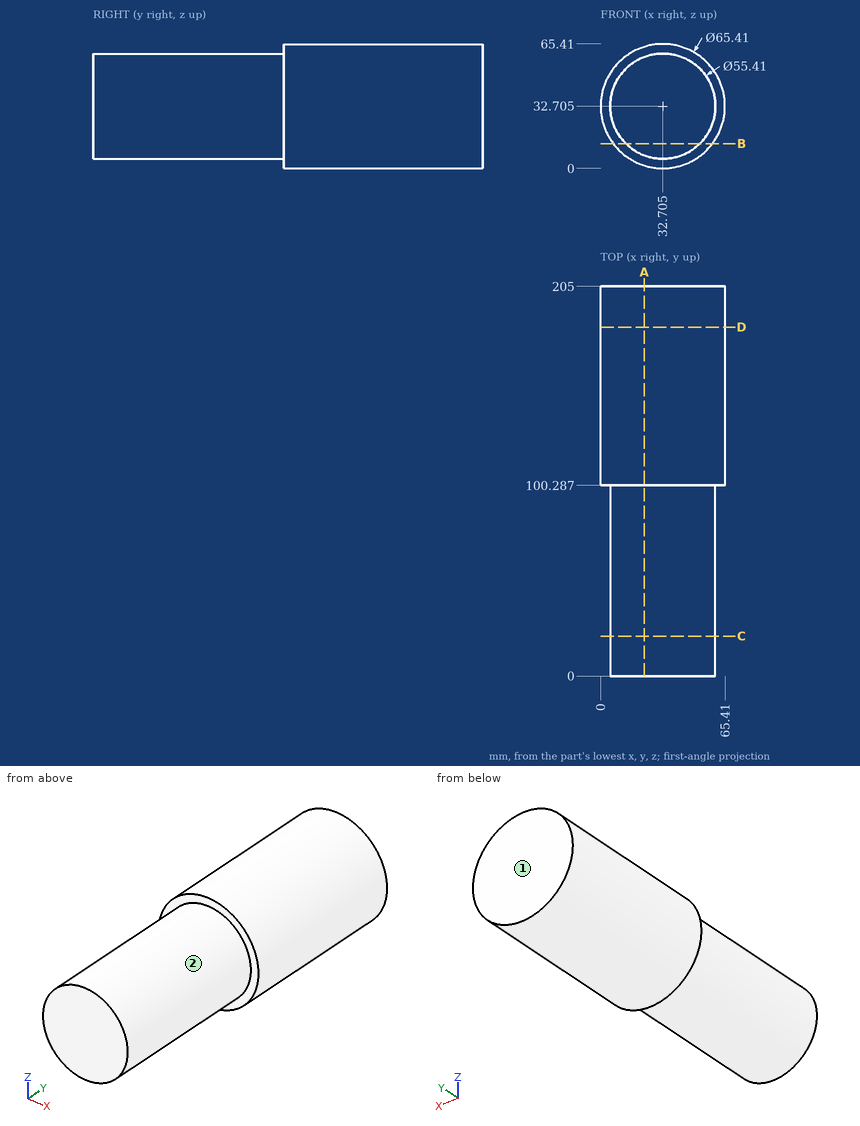
Study the drawing (mm; zero at the part's minimum x, y, z) and answer. A direction names the side the tool comes from. Round coordinates to 2 decimals unless told otherwise and drop trailing zeros. Write each loop counter-clockwise with the first axis right and the second up, starting at its lowest first coordinate (ties: lowest second). Pieces come first, ordered by that corner, then holes. Notation, with made-up numbers: (18, 27.25) - (39, 27.25) arc R13 cw to (39, 44.25) - close; hole circle Ø10 at (-37.5, 62). An arc over 180 degrees is marked (long way). Return JSON: item names as keys, results as strings. Group by question number.
Q1. The part is cut by section D-D on y = 183.5. Write down the section's boundary in (x, z) (3 decimals), then the cut area to 3 significant figures.
Q2. The part is cut by section B-B on z = 13. Write down the section's boundary in (x, y).
Q3. Each of these flat-tipped pins is pushed along its axis until it touches: pin 1 Ø4 at (y, z) = (46, 56.5) entering from -X; pin 2 Ø1 at (y, z) = (34, 58) entering from +X (1 decimal); pin 3 Ø5 at (x, y) = (20, 179.5) entering from +Z. Where does it stop, or does it pass through?
Q4. For the marked faces 1 and 2, determine the directions among +Z, -Z, +X, -X, +Y, -Y from which every point of the face is accessible in a straight line to the end or side of a thin tool.
Q5. The part is cut by section A-A on x = 23. Write down the section's boundary in (y, z), then the cut area to 3 significant figures.
Q6. Find the intervals of material crossed by L1, parallel to Z at x = 31.5, y = 125; L2, parallel to Y at x = 53, z = 54; L3, parallel to X at y = 191, z = 32, in increasing order.
Q7. The part is cut by section C-C on y = 21. Write down the section's boundary in (x, z) (3 decimals).
Solved:
{
 "1": {"outline": "circle Ø65.41 at (32.705, 32.705)", "area": "3,360 mm²"},
 "2": {"outline": "(6.6, 100.29) - (13.23, 100.29) - (13.23, 0) - (52.18, 0) - (52.18, 100.29) - (58.81, 100.29) - (58.81, 205) - (6.6, 205) - close"},
 "3": {"pin 1": "x = 15.6", "pin 2": "x = 45.1", "pin 3": "z = 63.78"},
 "4": {"face 1": "+Z, -Z, +X, -X, +Y", "face 2": "-Y"},
 "5": {"outline": "(0, 6.76) - (100.29, 6.76) - (100.29, 1.47) - (205, 1.47) - (205, 63.94) - (100.29, 63.94) - (100.29, 58.65) - (0, 58.65) - close", "area": "11,700 mm²"},
 "6": {"L1": "0.02 to 65.39", "L2": "100.29 to 205", "L3": "0.01 to 65.4"},
 "7": {"outline": "circle Ø55.41 at (32.705, 32.705)"}
}
